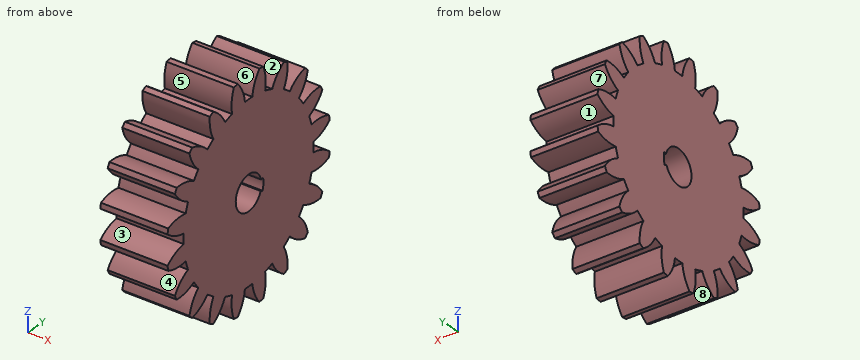
from build123d import *

# Parameters (mm, degrees)
BASPROSKE_W        = 10
BASPROSKE_H        = 16.5
TOOTHCUT_DEPTH     = 26.38700455
TEETHCUTS_COUNT    = 20
TEETHCUTS_ANGLE    = 342
BORSKE_R           = 2.5
BORE_DEPTH         = 50.0000508
CUT_EXTRUDE1_DEPTH = 26.197414545


with BuildPart() as part:
    # BasProSke → Base-Revolve (revolve)
    with BuildSketch(Plane(origin=(0, 0, 0), x_dir=(1, 0, 0), z_dir=(0, 1, 0)), mode=Mode.PRIVATE) as base_revolve_sk:
        with Locations((5, 8.25)):
            Rectangle(BASPROSKE_W, BASPROSKE_H)
    revolve(base_revolve_sk.sketch.rotate(Axis((-10, 0, 0), (1, 0, 0)), 180), axis=Axis((-10, 0, 0), (1, 0, 0)))

    # TooCutSke → ToothCut (cut, through all)
    with BuildSketch(Plane(origin=(0, 0, 0), x_dir=(0, 0, -1), z_dir=(1, 0, 0))):
        with BuildLine():
            ThreePointArc((0.74381438, 13.102904875), (0, 13.124), (-0.74381438, 13.102904875))
            ThreePointArc((-0.74381438, 13.102904875), (-1.226473103, 14.852072512), (-2.209965745, 16.376962373))
            ThreePointArc((-2.209965745, 16.376962373), (0, 16.5254), (2.209965745, 16.376962373))
            ThreePointArc((2.209965745, 16.376962373), (1.226473103, 14.852072512), (0.74381438, 13.102904875))
        make_face()
    toothcut = extrude(amount=TOOTHCUT_DEPTH, mode=Mode.SUBTRACT)

    # TeethCuts: ToothCut ×20 about axis
    teethcuts_axis = Axis((-10, 0, 0), (1, 0, 0))
    for i in range(1, TEETHCUTS_COUNT):
        add(toothcut.rotate(teethcuts_axis, i * TEETHCUTS_ANGLE / (TEETHCUTS_COUNT - 1)), mode=Mode.SUBTRACT)

    # BorSke → Bore (cut, symmetric)
    with BuildSketch(Plane(origin=(0, 0, 0), x_dir=(0, 0, -1), z_dir=(1, 0, 0))):
        with Locations(Location((0, 0, 0), (0, 0, 180))):
            Circle(BORSKE_R)
    extrude(amount=BORE_DEPTH, both=True, mode=Mode.SUBTRACT)

    # Sketch1 → Cut-Extrude1 (cut, through all)
    with BuildSketch(Plane.ZY):
        with BuildLine():
            Line((-1.07128416, 2.802204534), (-0.928446272, 2.428577263))
            ThreePointArc((-0.928446272, 2.428577263), (0.024935516, -2.599880424), (0.881694674, 2.445938368))
            ThreePointArc((0.881694674, 2.445938368), (0.758017697, 2.487048285), (0.63243603, 2.521908933))
            Line((0.63243603, 2.521908933), (0.729733881, 2.909894923))
            ThreePointArc((0.729733881, 2.909894923), (-0.179062708, 2.994651323), (-1.07128416, 2.802204534))
        make_face()
    extrude(amount=-CUT_EXTRUDE1_DEPTH, mode=Mode.SUBTRACT)


solid = part.part
Geometry check sheet. Reference: the model listing, model coordinates, mm. Face numbers are marked on the shaded views. A direction names the side the tool comes from. Round coordinates to 2 decimals unless told otherwise and drop trailing zeros. Write each loop counter-clockwise with the first axis right and the second up, starting at its lowest first coordinate (ties: lowest second). Pieces come first, ordered by that corner, then holes.
Item 1: Section check A-A (z = 0). Record the boundary of the cut face in (x, y), plus the area to 3 significant figures.
Determined:
outline: (0, -13.12) - (10, -13.12) - (10, -2.6) - (0, -2.6) - close; (0, 3) - (10, 3) - (10, 13.12) - (0, 13.12) - close
area: 206 mm2
Item 2: Material ranges on line 1 along Y through (x, z) = (4.25, 0); line 2 along Z through (x, y) = (7.25, 0); line 3 along Z through (x, y) = (7.5, 10.5), recorded low to high.
Determined:
line 1: y = -13.12 to -2.6, 3 to 13.12
line 2: z = -13.12 to -2.6, 2.6 to 13.12
line 3: z = -11.67 to -8.64, -7.87 to 7.87, 8.64 to 11.67
Item 3: Section check D-D (z = -6.5). Record the boundary of the cut face in (x, y), plus the area to 3 significant figures.
Determined:
outline: (0, -14.44) - (10, -14.44) - (10, 14.44) - (0, 14.44) - close
area: 289 mm2
Item 4: Access from +Z, -Z, +X, -X, +Y, -Y to the whole of each face (thin tool, end or side, straight path). Record for the marked faces 4, 5, 6, 7 and 8.
Determined:
face 4: +X, -X, -Y
face 5: +X, -X
face 6: +Z, +X, -X
face 7: +X, -X, +Y
face 8: -Z, +X, -X
Item 5: Section check C-C (y = -5.5). Record the boundary of the cut face in (x, z).
Determined:
outline: (0, -13.44) - (10, -13.44) - (10, 13.44) - (0, 13.44) - close
Item 6: Section check B-B (y = 0). Record the boundary of the cut face in (x, z).
Determined:
outline: (0, -13.12) - (10, -13.12) - (10, -2.6) - (0, -2.6) - close; (0, 2.6) - (10, 2.6) - (10, 13.12) - (0, 13.12) - close
Item 7: Go/stop test with flat-tipped pins: pin 1 Ø3 at (x, z) = (4, -5.5) entering from -Y; pin 2 Ø8 at (y, z) = (-9, -10) entering from -X; pin 3 Ø1.5 at (x, y) = (4.5, 10.5) entering from +Z; pin 4 Ø4 at (y, z) = (0, 0) entering from +X. Record where each tip stops, or that it passes through.
Determined:
pin 1: stops at y = -14.79
pin 2: stops at x = 0
pin 3: stops at z = 11.91
pin 4: passes through
Item 8: Mould release check, pull along Y, two halves, no side actions. Record for the marked faces 1, 2 and 3: +Y half, -Y half, draft (parallel to the pull), parting line (faces both ways), or undercut.
Determined:
face 1: +Y half
face 2: undercut
face 3: -Y half
